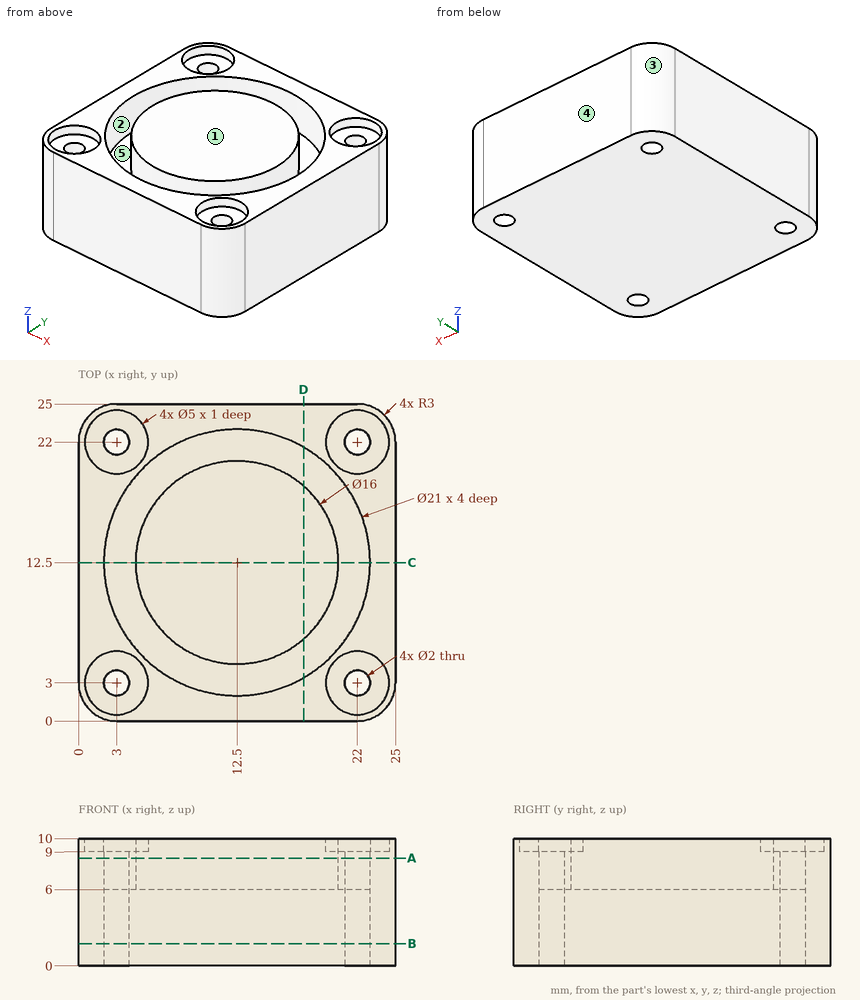
Source: three-view drawing plus pictorial views. Frame: mm from the lowest corner of the part. A direction names the side the tool comes from. Round coordinates to 2 decimals unless told otherwise and drop trailing zeros. Write each loop counter-clockwise with the first axis right and the second up, starting at its lowest first coordinate (ties: lowest second). Pieces come first, ordered by that corner, then holes. Notation, with made-up numbers: (-19, 80) -> (9, 80) arc R24 cw to (9, 119) -> close; hole circle Ø5 at (18.25, -27.5). An arc over 180 degrees is marked (long way). Return JSON: item names as keys, results as strings.
Q1. Section B-B on z = 1.75. Return the cut outline in (x, y).
From the geometry:
{"outline": "(0, 3) arc R3 ccw to (3, 0) -> (22, 0) arc R3 ccw to (25, 3) -> (25, 22) arc R3 ccw to (22, 25) -> (3, 25) arc R3 ccw to (0, 22) -> close; hole circle Ø2 at (3, 3); hole circle Ø2 at (3, 22); hole circle Ø2 at (22, 3); hole circle Ø2 at (22, 22)"}
Q2. Section C-C on y = 12.5. Return the cut outline in (x, z).
From the geometry:
{"outline": "(0, 0) -> (25, 0) -> (25, 10) -> (23, 10) -> (23, 6) -> (20.5, 6) -> (20.5, 10) -> (4.5, 10) -> (4.5, 6) -> (2, 6) -> (2, 10) -> (0, 10) -> close"}
Q3. First-contact query: pin 1 Ø3 at (x, y) = (22, 22) entering from +Z; pin 2 Ø1.6 at (x, y) = (3, 3) entering from +Z. Flat tips, straight axial feed; report the tip coordinate or a pass-through.
From the geometry:
{"pin 1": "z = 9", "pin 2": "through"}
Q4. Set-up query: the marked faces 4 and 5. Return all of +Z, -Z, +X, -X, +Y, -Y with unobstructed straight access to the full face (end or side cutting, diameter ignored); none if empty.
From the geometry:
{"face 4": "+Z, -Z, +X, -X, +Y", "face 5": "+Z"}
Q5. Section A-A on z = 8.5. Return the cut outline in (x, y), and give its area (3 significant figures).
From the geometry:
{"outline": "(0, 3) arc R3 ccw to (3, 0) -> (22, 0) arc R3 ccw to (25, 3) -> (25, 22) arc R3 ccw to (22, 25) -> (3, 25) arc R3 ccw to (0, 22) -> close; circle Ø16 at (12.5, 12.5); hole circle Ø2 at (3, 3); hole circle Ø21 at (12.5, 12.5); hole circle Ø2 at (3, 22); hole circle Ø2 at (22, 3); hole circle Ø2 at (22, 22)", "area": "459 mm2"}
Q6. Mould query, pull axis X, two halves, no side actions, for the marked faces 1, 2 and 3. Classes: +X half, -X half, draft (parallel to the pull), parting line (faces both ways), or undercut.
From the geometry:
{"face 1": "draft", "face 2": "undercut", "face 3": "-X half"}
Q7. Ray query, line 1 (X direction, y = 22, z = 3); line 2 (Y direction, x = 14.5, z = 9). Return the intervals inside material, ascending.
From the geometry:
{"line 1": "0 to 2, 4 to 21, 23 to 25", "line 2": "0 to 2.19, 4.75 to 20.25, 22.81 to 25"}
Q8. Section D-D on x = 17.75. Return the cut outline in (y, z), and give its area (3 significant figures).
From the geometry:
{"outline": "(0, 0) -> (25, 0) -> (25, 10) -> (21.59, 10) -> (21.59, 6) -> (18.54, 6) -> (18.54, 10) -> (6.46, 10) -> (6.46, 6) -> (3.41, 6) -> (3.41, 10) -> (0, 10) -> close", "area": "226 mm2"}
